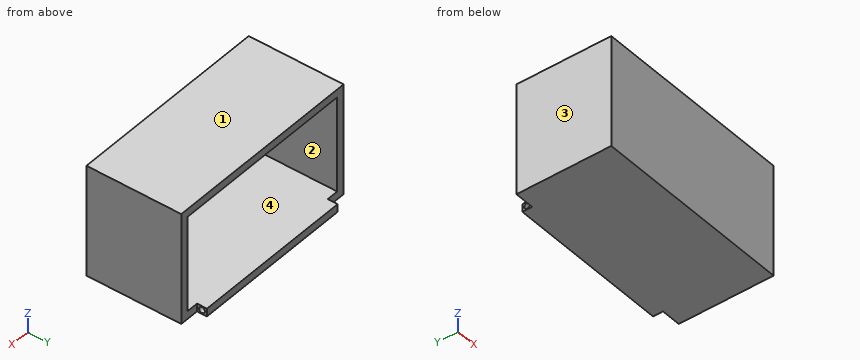
from build123d import *

# Parameters (mm, degrees)
SKETCH1_W           = 653.034
SKETCH1_H           = 304.8
BOSS_EXTRUDE1_DEPTH = 358.648
SHELL1_T            = -25.4
SKETCH2_W           = 526.034
SKETCH2_H           = 25.4
BOSS_EXTRUDE2_DEPTH = 31.75
SKETCH5_R           = 9.525
CUT_EXTRUDE2_DEPTH  = 25.4


with BuildPart() as part:
    # Sketch1 → Boss-Extrude1 (new body)
    with BuildSketch(Plane.XY):
        Rectangle(SKETCH1_W, SKETCH1_H)
    extrude(amount=BOSS_EXTRUDE1_DEPTH)

    # Shell1
    shell1_openings = [part.faces().sort_by_distance(p)[0] for p in [
        (0, 152.4, 179.324),
    ]]
    offset(amount=SHELL1_T, openings=shell1_openings, kind=Kind.INTERSECTION)

    # Sketch2 → Boss-Extrude2 (add)
    with BuildSketch(Plane(origin=(0, 152.4, 0), x_dir=(1, 0, 0), z_dir=(0, 1, 0))):
        with Locations((0, -12.7)):
            Rectangle(SKETCH2_W, SKETCH2_H)
    extrude(amount=BOSS_EXTRUDE2_DEPTH)

    # Sketch5 → Cut-Extrude2 (cut)
    with BuildSketch(Plane(origin=(263.017, 0, 0), x_dir=(0, 0, -1), z_dir=(1, 0, 0))):
        with Locations((-12.7, 168.275)):
            Circle(SKETCH5_R)
    cut_extrude2 = extrude(amount=-CUT_EXTRUDE2_DEPTH, mode=Mode.SUBTRACT)

    # Mirror2: Cut-Extrude2 across plane
    add(cut_extrude2.mirror(Plane(origin=(0, 0, 0), x_dir=(0, 0, 1), z_dir=(1, 0, 0))), mode=Mode.SUBTRACT)


solid = part.part
Work out the finished part from the listing and answer in its coordinate system (mm). Face numbers are marked on the shaded views. Coordinates: 2 decimals unless noted, no trailing zeros. Write each loop counter-clockwise with the first axis right and the second up, starting at its lowest first coordinate (ties: lowest second). Pieces come first, ordered by that corner, then holes. Notation, with made-up numbers: M -33.5,2 L -20.5,2 A27 cw -20.5,22 Z; hole C 27.25,71.25 d9. An arc over 180 degrees is marked long. Use one line per item in the form item = value. Start each with the question number.
1. Straight lines are drawn through the part: probe 1 along X at (y, z) = (96, 246.5); probe 2 along Y at (x, z) = (-258, 12.7); probe 3 along Z at (x, y) = (80, -32). For each, find the intervals that lie inside material, in ascending order. Write a range as from..to.
2. The mould has two halves that part along X. Classify the marked faces 1, 2, 3 and 4: released by +X, released by -X, zero draft, split by the parting line, or undercut.
3. The part is cut by section B-B (x = 196). Give the vertices of the cut face in (y, z).
4. Each of these flat-tipped pins is pushed along its axis until it touches: P1, Ø11.5, axis at y = 168.275, z = 12.7, coming from the -X side; P2, Ø12.5, axis at y = 176, z = 10, coming from the -X side; P3, Ø17, axis at y = 168.275, z = 12.7, coming from the +X side. Where does it stop, or does it pass through?
5. The part is cut by section D-D (z = 220). Give the vertices of the cut face in (x, y), plus the area to 3 significant figures.
6. The part is cut by section A-A (y = 71). Give the vertices of the cut face in (x, z).
7. The part is cut by section C-C (z = 12.7). Give the vertices of the cut face in (x, y).
Evaluation:
q1.probe_1 = -326.52..-301.12, 301.12..326.52
q1.probe_2 = -152.4..158.75, 177.8..184.15
q1.probe_3 = 0..25.4, 333.25..358.65
q2.face_1 = zero draft
q2.face_2 = undercut
q2.face_3 = released by -X
q2.face_4 = undercut
q3.outline = M -152.4,0 L 184.15,0 L 184.15,25.4 L -127,25.4 L -127,333.25 L 152.4,333.25 L 152.4,358.65 L -152.4,358.65 Z
q4.P1 = -237.62
q4.P2 = -263.02
q4.P3 = 237.62
q5.outline = M -326.52,-152.4 L 326.52,-152.4 L 326.52,152.4 L 301.12,152.4 L 301.12,-127 L -301.12,-127 L -301.12,152.4 L -326.52,152.4 Z
q5.area = 30,800 mm^2
q6.outline = M -326.52,0 L 326.52,0 L 326.52,358.65 L -326.52,358.65 Z; hole M -301.12,25.4 L 301.12,25.4 L 301.12,333.25 L -301.12,333.25 Z
q7.outline = M -326.52,-152.4 L 326.52,-152.4 L 326.52,152.4 L 263.02,152.4 L 263.02,158.75 L 237.62,158.75 L 237.62,177.8 L 263.02,177.8 L 263.02,184.15 L -263.02,184.15 L -263.02,177.8 L -237.62,177.8 L -237.62,158.75 L -263.02,158.75 L -263.02,152.4 L -326.52,152.4 Z
